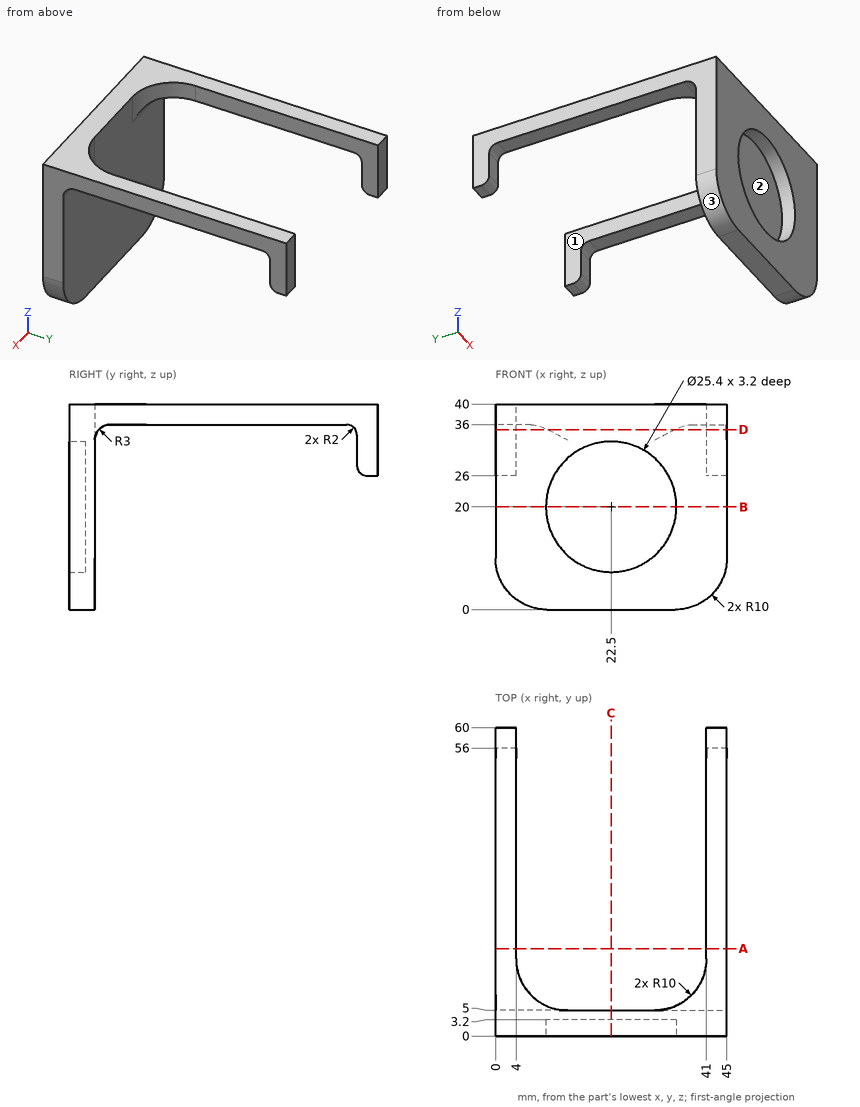
Print and shaded views of the part. All mm, measured from the part's lowest x, y and z. A direction names the side the tool comes from. Give positions to 0.01 mm unless a question says otherwise; leave off trailing zeros. Loops run counter-clockwise (first coordinate to the right, second up) from the corner with the lowest first, then second, coordinate; pieces in that order, holes last. Notation, with made-up numbers: (39, 4.5) -> (74, 4.5) arc R20 ccw to (74, 43.5) -> close; hole circle Ø2 at (34.5, -28.75). An arc over 180 degrees is marked (long way). One line per question, with ' | ' between items. Start each with the question number.
1) Probe L1, parallel to X at y = 1, z = 20; L2, parallel to Z at x = 22, y = 2; L3, parallel to Y at x = 16, z = 35. List the from-to ranges inside material, lowest first.
2) Cut at B-B (z = 20). Give the cut face in (x, y), plus the area to 3 significant figures.
3) Cut at D-D (z = 35). Give the cut face in (x, y).
4) Cut at A-A (y = 17). Give the cut face in (x, z), plus the area to 3 significant figures.
5) 3-axis set-ups, long thin cutter, end or side, ignore diameter. For the marked faces 1, 2 and 3: which of +Z, -Z, +X, -X, +Y, -Y reach the whole face in a straight line?
6) Cut at C-C (x = 22.5). Give the cut face in (y, z), plus the area to 3 significant figures.
7) Pin check, flat tips, straight feed: pin 1 (5.5 mm diameter, centred on x = 3, y = 39.5, fed in from -Z); pin 2 (5 mm diameter, centred on x = 21, z = 28.5, fed in from -Y); pin 3 (1.6 mm diameter, centred on x = 2, y = 58.5, fed in from -Z). Stop position of each tip, or through.
Return value:
1) L1: 0 to 9.8, 35.2 to 45 | L2: 0 to 7.31, 32.69 to 40 | L3: 0 to 5
2) outline: (0, 0) -> (9.8, 0) -> (9.8, 3.2) -> (35.2, 3.2) -> (35.2, 0) -> (45, 0) -> (45, 5) -> (0, 5) -> close | area: 144 mm^2
3) outline: (0, 0) -> (45, 0) -> (45, 5.76) -> (34.83, 5.76) arc R10 cw to (31, 5) -> (14, 5) arc R10 cw to (10.17, 5.76) -> (0, 5.76) -> close; (0, 55.73) -> (4, 55.73) -> (4, 60) -> (0, 60) -> close; (41, 55.73) -> (45, 55.73) -> (45, 60) -> (41, 60) -> close
4) outline: (0, 36) -> (4, 36) -> (4, 40) -> (0, 40) -> close; (41, 36) -> (45, 36) -> (45, 40) -> (41, 40) -> close | area: 32.0 mm^2
5) face 1: +Z, -Z, +Y | face 2: -Y | face 3: -Z, -X, +Y, -Y
6) outline: (0, 0) -> (5, 0) -> (5, 40) -> (0, 40) -> (0, 32.7) -> (3.2, 32.7) -> (3.2, 7.3) -> (0, 7.3) -> close | area: 119 mm^2
7) pin 1: z = 36 | pin 2: y = 3.2 | pin 3: z = 26
